```python
from build123d import *

# Parameters (mm, degrees)
SKETCH1_R           = 45
SKETCH1_R_2         = 2
SKETCH1_R_3         = 2.5
SKETCH1_W           = 20.2
SKETCH1_H           = 40.5
BOSS_EXTRUDE1_DEPTH = 5
CUT_EXTRUDE1_DEPTH  = 10


with BuildPart() as part:
    # Sketch1 → Boss-Extrude1 (new body)
    with BuildSketch(Plane.XY):
        Circle(SKETCH1_R)
        with Locations((0, 42.5)):
            Circle(SKETCH1_R_2, mode=Mode.SUBTRACT)
        with Locations((-42.5, 0)):
            Circle(SKETCH1_R_2, mode=Mode.SUBTRACT)
        with Locations((0, -42.5)):
            Circle(SKETCH1_R_2, mode=Mode.SUBTRACT)
        with Locations((42.5, 0)):
            Circle(SKETCH1_R_2, mode=Mode.SUBTRACT)
        with Locations((-5, -13.85)):
            Circle(SKETCH1_R_3, mode=Mode.SUBTRACT)
        with Locations((5, -13.85)):
            Circle(SKETCH1_R_3, mode=Mode.SUBTRACT)
        with Locations((5, 34.15)):
            Circle(SKETCH1_R_3, mode=Mode.SUBTRACT)
        with Locations((-5, 34.15)):
            Circle(SKETCH1_R_3, mode=Mode.SUBTRACT)
        with Locations((0, 10.15)):
            Rectangle(SKETCH1_W, SKETCH1_H, mode=Mode.SUBTRACT)
    extrude(amount=BOSS_EXTRUDE1_DEPTH)

    # Sketch2 → Cut-Extrude1 (cut)
    with BuildSketch(Plane.XY.offset(5)):
        with BuildLine():
            Line((27, 18), (27, -8))
            ThreePointArc((27, -8), (23, -12), (19, -8))
            Line((19, -8), (19, 18))
            ThreePointArc((19, 18), (23, 22), (27, 18))
        make_face()
    extrude(amount=-CUT_EXTRUDE1_DEPTH, mode=Mode.SUBTRACT)


solid = part.part
```
The model under review builds one solid part; all positions refer to its coordinate system, in mm. Round coordinates to 2 decimals unless told otherwise and drop trailing zeros. Loops run counter-clockwise (first coordinate to the right, second up) from the corner with the lowest first, then second, coordinate; pieces in that order, holes last. Notation, with made-up numbers: (81, 1.5) - (109, 1.5) arc R15 ccw to (109, 10.5) - close; hole circle Ø7 at (3, 52). An arc over 180 degrees is marked (long way). Use a Markdown table: item, result. Add a question column.
Q1. Add section C-C (y = 34.15). State the section outline as (x, z) points, plus the area to 3 significant figures.
Q2. Insertion check: pin 1 Ø2.5 at (y, z) = (5, 3) entering from -X; pin 2 Ø1 at (x, z) = (-17.5, 3.5) entering from -Y; pin 3 Ø2.5 at (x, z) = (-1.5, 3) entering from +Y. Each pin has a flat end and moves straight along its axis. Give the tip position at first contact, or say it passes through.
Q3. Add section D-D (x = 42.5). State the section outline as (y, z) points.
Q4. Add section B-B (z = 1.65). State how many separate pieces and enclosed holes the cut face has, plus the area to 3 significant figures.
Q5. For probe 1 along Y at (x, z) = (0, 1.65); probe 2 along X at (y, z) = (13.5, 3.25); probe 3 along Y at (x, z) = (5, 2.55), list the stretches that pass through material, from the lowest coordinate up.
Q6. The part is to be moulded in two halves that separate along Y. For faces 1 (the face through (20.765, -39.923, 2.465)), 2 (the face through (-11, 1, 5)), 3 (the face through (-0.434, 40.548, 2.465)), say which applies: pulls with the +Y half, pulls with the -Y half, needs draft (parallel to the pull), parting line crosses it, or undercut.
Q7. Add section A-A (x = 5). State the section outline as (y, z) points, plus the area to 3 significant figures.
Worked answers:
| question | item | result |
|---|---|---|
| 1 | outline | (-29.3, 0) - (-7.5, 0) - (-7.5, 5) - (-29.3, 5) - close; (-2.5, 0) - (2.5, 0) - (2.5, 5) - (-2.5, 5) - close; (7.5, 0) - (29.3, 0) - (29.3, 5) - (7.5, 5) - close |
| 1 | area | 243 mm² |
| 2 | pin 1 | x = -44.84 |
| 2 | pin 2 | y = -41.67 |
| 2 | pin 3 | y = 45 |
| 3 | outline | (-14.79, 0) - (-2, 0) - (-2, 5) - (-14.79, 5) - close; (2, 0) - (14.79, 0) - (14.79, 5) - (2, 5) - close |
| 4 | separate pieces | 1 |
| 4 | enclosed holes | 10 |
| 4 | area | 5,160 mm² |
| 5 | probe 1 | -45 to -44.5, -40.5 to -10.1, 30.4 to 40.5, 44.5 to 45 |
| 5 | probe 2 | -42.93 to -10.1, 10.1 to 19, 27 to 42.93 |
| 5 | probe 3 | -44.72 to -16.35, -11.35 to -10.1, 30.4 to 31.65, 36.65 to 44.72 |
| 6 | face 1 | parting line crosses it |
| 6 | face 2 | needs draft |
| 6 | face 3 | undercut |
| 7 | outline | (-44.72, 0) - (-16.35, 0) - (-16.35, 5) - (-44.72, 5) - close; (-11.35, 0) - (-10.1, 0) - (-10.1, 5) - (-11.35, 5) - close; (30.4, 0) - (31.65, 0) - (31.65, 5) - (30.4, 5) - close; (36.65, 0) - (44.72, 0) - (44.72, 5) - (36.65, 5) - close |
| 7 | area | 195 mm² |
